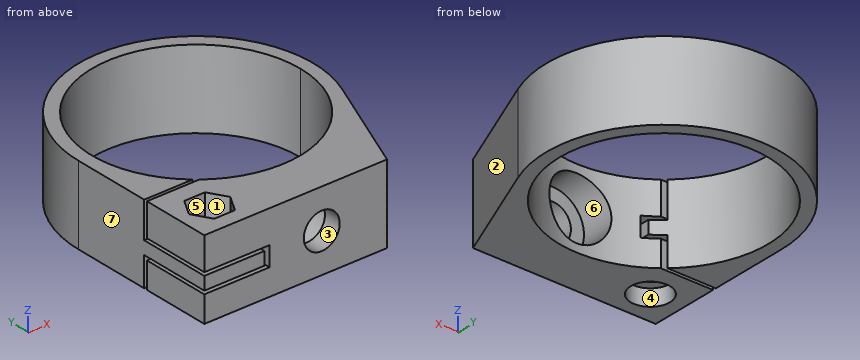
```python
from build123d import *

# Parameters (mm, degrees)
F0_R          = 16
F1_DEPTH      = 6
F1_DEPTH_BACK = 6
F4_DEPTH      = 25
F5_W          = 0.5
F5_H          = 4
F5_H_2        = 5
F6_DEPTH      = 8.0135078223
F8_D          = 3
F9_DEPTH      = 3.5
F10_R         = 3
F11_DEPTH     = 2.5
F13_D         = 5.5
F13_DEPTH     = 23.001
F14_R         = 4.75
F15_DEPTH     = 20.3


with BuildPart() as f1:
    # F0 (on Top) → F1 (new body, two sides)
    with BuildSketch(Plane.XY) as f1_sk:
        with BuildLine():
            Line((10, -23), (16.6457856397, -6.8496584175))
            ThreePointArc((16.6457856397, -6.8496584175), (3.4911214878, 17.6582012322), (-18, 0))
            Line((-18, 0), (-18, -23))
            Line((-18, -23), (10, -23))
        make_face()
        Circle(F0_R, mode=Mode.SUBTRACT)
    extrude(amount=F1_DEPTH)
    extrude(f1_sk.sketch, amount=-F1_DEPTH_BACK)

    # F3 (on offset) → F4 (cut)
    with BuildSketch(Plane.XZ.offset(12)):
        Polygon((-8.8, -1.5), (-18, -1.5), (-18, -2), (-8, -2), (-8, 1), (-18, 1), (-18, 0.5), (-8.8, 0.5), align=None)
    extrude(amount=F4_DEPTH, mode=Mode.SUBTRACT)

    # F5 (on face) → F6 (cut, through all)
    with BuildSketch(Plane(origin=(-18, 0, 0), x_dir=(0, -1, 0), z_dir=(-1, 0, 0))):
        with Locations((12.25, -4)):
            Rectangle(F5_W, F5_H)
        with Locations((12.25, 3.5)):
            Rectangle(F5_W, F5_H_2)
    extrude(amount=-F6_DEPTH, mode=Mode.SUBTRACT)

    # F8 (through all)
    with Locations(Plane.XY.offset(6)):
        with Locations((-13, -18)):
            Hole(F8_D / 2)

    # F7 (on face) → F9 (cut)
    with BuildSketch(Plane.XY.offset(6)):
        Polygon((-11.4122867597, -20.75), (-9.8245735195, -18), (-11.4122867597, -15.25), (-14.5877132403, -15.25), (-16.1754264805, -18), (-14.5877132403, -20.75), align=None)
    extrude(amount=-F9_DEPTH, mode=Mode.SUBTRACT)

    # F10 (on face) → F11 (cut)
    with BuildSketch(Plane(origin=(0, 0, -6), x_dir=(1, 0, 0), z_dir=(0, 0, -1))):
        with Locations((-13, 18)):
            Circle(F10_R)
    extrude(amount=-F11_DEPTH, mode=Mode.SUBTRACT)

    # F13 (through all, one way)
    with BuildSketch(Plane(origin=(0, 0, 0), x_dir=(1, 0, 0), z_dir=(0, 1, 0))):
        with Locations((0, 0)):
            Circle(F13_D / 2)
    extrude(amount=-F13_DEPTH, mode=Mode.SUBTRACT)

    # F14 (on Front) → F15 (cut)
    with BuildSketch(Plane.XZ):
        Circle(F14_R)
    extrude(amount=F15_DEPTH, mode=Mode.SUBTRACT)


solid = f1.part
```
The model under review builds one solid part; all positions refer to its coordinate system, in mm. Face numbers are marked on the shaded views. A direction names the side the tool comes from. Coordinates: 2 decimals unless noted, no trailing zeros. Write each loop counter-clockwise with the first axis right and the second up, starting at its lowest first coordinate (ties: lowest second). Pieces come first, ordered by that corner, then holes.
1) Clearance check with flat-ended pins moving along their axes: pin 1 Ø5.5 at (x, z) = (-12.5, 4.5) entering from +Y; pin 2 Ø5 at (x, y) = (-13, -18) entering from -Z; pin 3 Ø2.5 at (x, y) = (-13, -18) entering from -Z; pin 4 Ø1.6 at (x, z) = (-13, 3.5) entering from +Y. State where each tip first meets the part, or that it passes through.
2) We need section C-C on y = -17.5. Count the separate pieces of the cut face and the enclosed holes in it, then the cut area to 3 significant figures.
3) We need section A-A on z = -1. State the section outline as (x, y) points, then the cut area to 3 significant figures.
4) We need section D-D on x = 8. State the section outline as (y, z) points.
5) The part is to be moulded in two halves that separate along Y. For the marked faces 1, 2, 3 and 4, say which applies: pulls with the +Y half, pulls with the -Y half, needs draft (parallel to the pull), parting line crosses it, or undercut.
6) To check wall thickness, follow probe 1 along Y at (x, z) = (0, 3.75); probe 2 along Z at (x, y) = (0, -17); probe 3 along Y at (x, z) = (-13, -4.9). State the ranges of each line that lie inside material, in increasing order.
7) Machinability: for the marked faces 5, 6 and 7, which of the approach directions +Z, -Z, +X, -X, +Y, -Y give a long, thin tool a straight path to every point of the face, cutting with its end or side? Answer none if there is none.
8) We need section B-B on x = 0. State the section outline as (y, z) points.
Answer list:
1. pin 1: stops at y = 15.13
1. pin 2: stops at z = -3.5
1. pin 3: passes through
1. pin 4: stops at y = 13.23
2. separate pieces: 5
2. enclosed holes: 1
2. area: 232 mm2
3. outline: (-18, -23) - (-8.8, -23) - (-8.8, -13.36) arc R16 cw (long way) to (4.64, -15.31) - (4.64, -20.3) - (2.56, -20.3) - (2.56, -23) - (10, -23) - (16.65, -6.85) arc R18 ccw (long way) to (-18, 0) - close; (-8, -23) - (-2.56, -23) - (-2.56, -20.3) - (-4.64, -20.3) - (-4.64, -15.31) arc R16 cw to (-8, -13.86) - close; hole circle Ø3 at (-13, -18)
3. area: 384 mm2
4. outline: (-23, -6) - (-13.86, -6) - (-13.86, 6) - (-23, 6) - close; (13.86, -6) - (16.12, -6) - (16.12, 6) - (13.86, 6) - close
5. face 1: undercut
5. face 2: pulls with the -Y half
5. face 3: needs draft
5. face 4: undercut
6. probe 1: y = -23 to -20.3, 16 to 18
6. probe 2: z = -6 to -4.75, 4.75 to 6
6. probe 3: y = -23 to -21, -15 to -12.5, -12 to -9.33, 9.33 to 12.45
7. face 5: +Z
7. face 6: none
7. face 7: +Z, -Z, -X, +Y, -Y
8. outline: (-23, -6) - (-16, -6) - (-16, -4.75) - (-20.3, -4.75) - (-20.3, -2.75) - (-23, -2.75) - close; (-23, 2.75) - (-20.3, 2.75) - (-20.3, 4.75) - (-16, 4.75) - (-16, 6) - (-23, 6) - close; (16, -6) - (18, -6) - (18, 6) - (16, 6) - close
